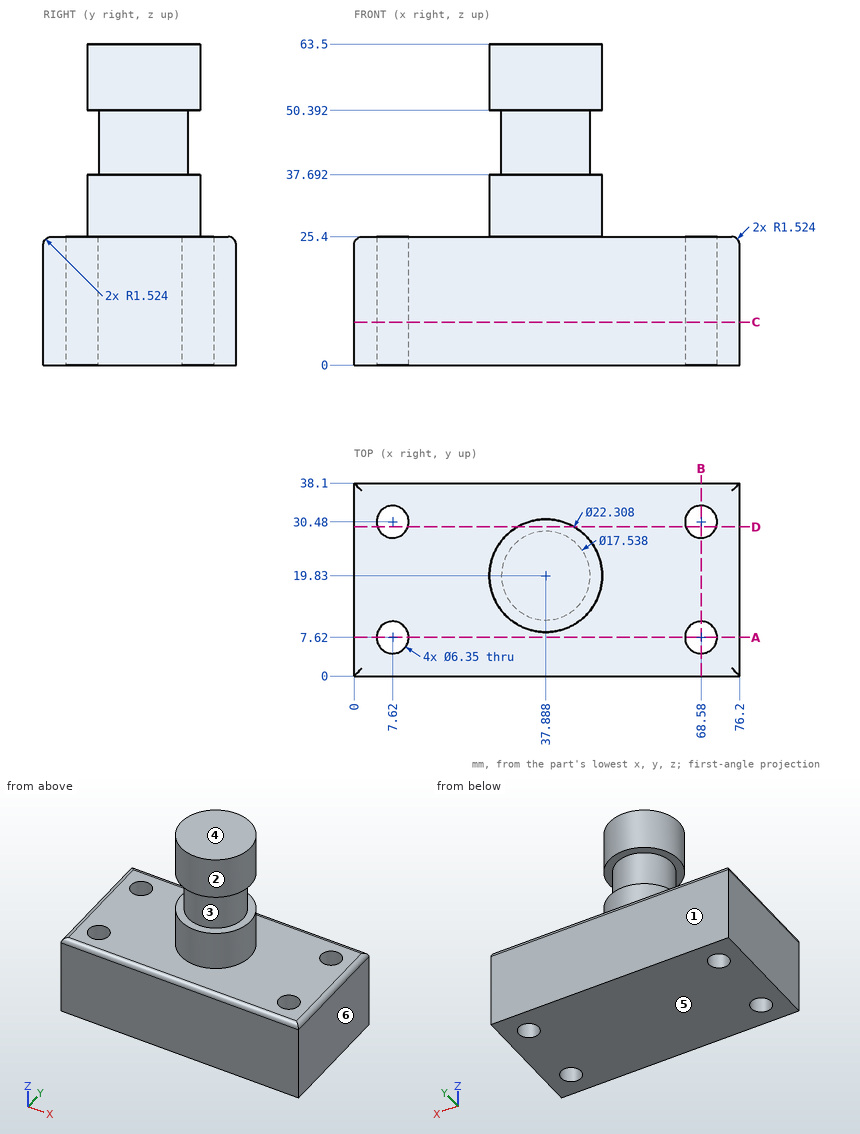
Check sheet for the drawn part. Datum: minimum x, y, z corner. Units: mm. A direction names the side the tool comes from. Coordinates: 2 decimals unless noted, no trailing zeros. Order: outer loops, then holes, each group sorted by start corner. A loop starts at its lowest first (then second) coordinate and runs counter-clockwise, first axis right, second up. Notation, with made-up numbers: (59, -39.5) -> (68, -39.5) arc R31 ccw to (68, -4.5) -> close; hole circle Ø1 at (31, 53.5). An arc over 180 degrees is marked (long way). Use a Markdown table: item, result. Add a question column.
1. Cross-section at A-A (y = 7.62). Enter the section's corners in (x, z) (1 decimal).
2. Material ranges on L1, parallel to Y at x = 7.62, z = 19 (1 decimal); L2, parallel to X at y = 30, z = 7; L3, parallel to Z at x = 43.5, y = 28, recorded low to high.
3. Cross-section at C-C (z = 8.5). Give the number of separate pieces and of enclosed holes in the cut face, and give its area (3 significant figures).
4. Go/stop test with flat-tipped pins: pin 1 Ø5 at (y, z) = (18.5, 52) entering from -X; pin 2 Ø1.5 at (y, z) = (21, 48) entering from -X; pin 3 Ø6 at (x, z) = (43.5, 56.5) entering from +Y. Record where each tip stops, or that it passes through.
5. Cross-section at B-B (x = 68.58). Enter the section's corners in (y, z) (1 decimal), and give its area (3 significant figures).
6. Cross-section at D-D (y = 29.5). Enter the section's corners in (x, z), and give its area (3 significant figures).
7. Set-up check for the marked faces 1 and 2: record each of +Z, -Z, +X, -X, +Y, -Y from which the full face is reachable in a straight line by a thin tool's end or side.
8. Mould release check, pull along Z, two halves, no side actions. Record for the marked faces 3, 4, 5 and 6: pulls with the +Z half, pulls with the -Z half, needs draft (parallel to the pull), parting line crosses it, or undercut.
Filled sheet:
| question | item | result |
|---|---|---|
| 1 | outline | (0, 0) -> (4.4, 0) -> (4.4, 25.4) -> (1.5, 25.4) arc R1.5 ccw to (0, 23.9) -> close; (10.8, 0) -> (65.4, 0) -> (65.4, 25.4) -> (10.8, 25.4) -> close; (71.8, 0) -> (76.2, 0) -> (76.2, 23.9) arc R1.5 ccw to (74.7, 25.4) -> (71.8, 25.4) -> close |
| 2 | L1 | 0 to 4.4, 10.8 to 27.3, 33.7 to 38.1 |
| 2 | L2 | 0 to 4.48, 10.76 to 65.44, 71.72 to 76.2 |
| 2 | L3 | 0 to 37.69, 50.39 to 63.5 |
| 3 | separate pieces | 1 |
| 3 | enclosed holes | 4 |
| 3 | area | 2,780 mm2 |
| 4 | pin 1 | x = 26.73 |
| 4 | pin 2 | x = 29.13 |
| 4 | pin 3 | y = 30.67 |
| 5 | outline | (0, 0) -> (4.4, 0) -> (4.4, 25.4) -> (1.5, 25.4) arc R1.5 ccw to (0, 23.9) -> close; (10.8, 0) -> (27.3, 0) -> (27.3, 25.4) -> (10.8, 25.4) -> close; (33.7, 0) -> (38.1, 0) -> (38.1, 23.9) arc R1.5 ccw to (36.6, 25.4) -> (33.7, 25.4) -> close |
| 5 | area | 644 mm2 |
| 6 | outline | (0, 0) -> (4.6, 0) -> (4.6, 25.4) -> (1.52, 25.4) arc R1.52 ccw to (0, 23.88) -> close; (10.64, 0) -> (65.56, 0) -> (65.56, 25.4) -> (43.45, 25.4) -> (43.45, 37.69) -> (32.33, 37.69) -> (32.33, 25.4) -> (10.64, 25.4) -> close; (32.33, 50.39) -> (43.45, 50.39) -> (43.45, 63.5) -> (32.33, 63.5) -> close; (71.6, 0) -> (76.2, 0) -> (76.2, 23.88) arc R1.52 ccw to (74.68, 25.4) -> (71.6, 25.4) -> close |
| 6 | area | 1,910 mm2 |
| 7 | face 1 | +Z, -Z, +X, -X, +Y |
| 7 | face 2 | +Z |
| 8 | face 3 | undercut |
| 8 | face 4 | pulls with the +Z half |
| 8 | face 5 | pulls with the -Z half |
| 8 | face 6 | needs draft |
